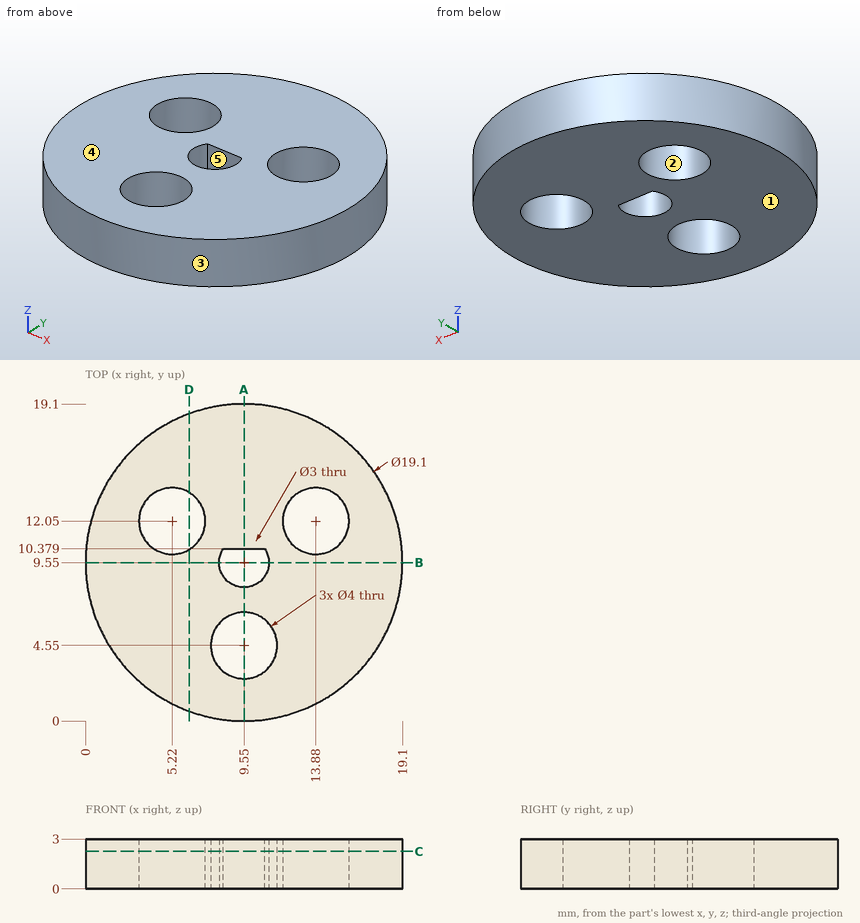
For this review, use the dimensioned drawing (mm, ordinates from the lowest corner) and the shaded views. A direction names the side the tool comes from. Round coordinates to 2 decimals unless told otherwise and drop trailing zeros. Order: outer loops, then holes, each group sorted by start corner. A loop starts at its lowest first (then second) coordinate and runs counter-clockwise, first axis right, second up. Notation, with made-up numbers: (62.5, 30) -> (76.5, 30) arc R28 cw to (76.5, 66) -> close; hole circle Ø6 at (39, 46). An arc over 180 degrees is marked (long way). One line per item, written item: value. Start each with the question number.
Q1. Take a section at D-D (x = 6.25). Write out the cut boundary in (y, z), and give its area (3 significant figures).
Q2. Take a section at B-B (y = 9.55). Write out the cut boundary in (x, z), and give its area (3 significant figures).
Q3. Clearance check with flat-ended pins moving along their axes: pin 1 Ø3.5 at (x, y) = (9.55, 4.55) entering from +Z; pin 2 Ø1.5 at (y, z) = (15.5, 1.5) entering from +X; pin 3 Ø1 at (x, z) = (7.5, 1.5) entering from +Y; pin 4 Ø6.5 at (x, y) = (5.22, 12.05) entering from +Z. State where each tip first meets the part, or that it passes through.
Q4. Machinability: for the marked faces 4 and 5, which of the approach directions +Z, -Z, +X, -X, +Y, -Y give a long, thin tool a straight path to every point of the face, cutting with its end or side? Answer none if there is none.
Q5. Take a section at A-A (x = 9.55). Write out the cut boundary in (y, z).
Q6. Mouldability with a two-part tool opening along X and no side actions: class the marked faces 1, 2 and 3 as released by +X, released by -X, zero draft, split by the parting line, or undercut.
Q7. Take a section at C-C (z = 2.25). Write out the cut boundary in (x, y).
Q8. Wall thickness on line 1 (Y direction, x = 9.55, z = 1.85); line 2 (X direction, y = 12.75, z = 1.8); line 3 (Y direction, x = 10.25, z = 2.9): over which ranges is each line inside the solid? List them lowest first.
Reported:
1. outline: (0.59, 0) -> (10.34, 0) -> (10.34, 3) -> (0.59, 3) -> close; (13.76, 0) -> (18.51, 0) -> (18.51, 3) -> (13.76, 3) -> close
1. area: 43.5 mm2
2. outline: (0, 0) -> (8.05, 0) -> (8.05, 3) -> (0, 3) -> close; (11.05, 0) -> (19.1, 0) -> (19.1, 3) -> (11.05, 3) -> close
2. area: 48.3 mm2
3. pin 1: passes through
3. pin 2: stops at x = 17.56
3. pin 3: stops at y = 18.97
3. pin 4: stops at z = 3
4. face 4: +Z, +X, -X, +Y, -Y
4. face 5: +Z, -Z
5. outline: (0, 0) -> (2.55, 0) -> (2.55, 3) -> (0, 3) -> close; (6.55, 0) -> (8.05, 0) -> (8.05, 3) -> (6.55, 3) -> close; (10.38, 0) -> (19.1, 0) -> (19.1, 3) -> (10.38, 3) -> close
6. face 1: zero draft
6. face 2: undercut
6. face 3: split by the parting line
7. outline: circle Ø19.1 at (9.55, 9.55); hole circle Ø4 at (5.22, 12.05); hole circle Ø4 at (9.55, 4.55); hole (8.3, 10.38) arc R1.5 ccw (long way) to (10.8, 10.38) -> close; hole circle Ø4 at (13.88, 12.05)
8. line 1: y = 0 to 2.55, 6.55 to 8.05, 10.38 to 19.1
8. line 2: x = 0.55 to 3.35, 7.09 to 12.01, 15.75 to 18.55
8. line 3: y = 0.03 to 2.68, 6.42 to 8.22, 10.38 to 19.07
